from build123d import *

# Parameters (mm, degrees)
BOSS_EXTRUDE1_DEPTH = 3


with BuildPart() as part:
    # Sketch1 → Boss-Extrude1 (new body)
    with BuildSketch(Plane(origin=(0, 0, 0), x_dir=(1, 0, 0), z_dir=(0, 1, 0))):
        Polygon((-5, 44.5), (-25.5, 35.5), (25.5, 35.5), (5, 44.5), align=None)
        Polygon((-25.5, 35.5), (-35.5, 35.5), (-35.5, -35.5), (35.5, -35.5), (35.5, 35.5), (25.5, 35.5), align=None)
    extrude(amount=BOSS_EXTRUDE1_DEPTH)


solid = part.part
Design review of the part built by this model. Coordinates are the model's own, in mm. A direction names the side the tool comes from. Coordinates: 2 decimals unless noted, no trailing zeros. Loops run counter-clockwise (first coordinate to the right, second up) from the corner with the lowest first, then second, coordinate; pieces in that order, holes last. Notation, with made-up numbers: (-31.5, 22) - (-12.5, 22) arc R13 cw to (-12.5, 31) - close; hole circle Ø2 at (56.25, 56). An arc over 180 degrees is marked (long way). Use CSV: the item, a comma, the result in double quotes. Start each with the question number.
1. Add section C-C on z = -38. Give the boundary of the cut face in (x, y), plus the area to 3 significant figures.
2. Clearance check with a flat-ended pin moving along its axis: pin 1 (1.5 mm diameter, centred on x = -29, y = 2, fed in from -Z). State where the tip first meets the part, or that it passes through.
3. Add section A-A on y = 1.2. Give the boundary of the cut face in (x, z), plus the area to 3 significant figures.
4. For faces 1 (the flat face through (0, 3, -5)), 2 (the flat face through (-30, 1, -35.5)), 3 (the flat face through (31, 1, -35.5)), list the 3-axis set-ups (+Z, -Z, +X, -X, +Y, -Y) from which the entire face can be reached by the end or side of a thin tool; tool diameter is ignored.
5. Add section B-B on x = 10. Give the boundary of the cut face in (y, z).
6. To check wall thickness, follow probe 1 along Z at (x, y) = (-32, 1.95); probe 2 along Z at (x, y) = (9, 1.5); probe 3 along X at (y, z) = (0.95, -36). State the ranges of each line that lie inside material, in increasing order.
Resolved:
1,outline,"(-19.81, 0) - (19.81, 0) - (19.81, 3) - (-19.81, 3) - close"
1,area,"119 mm2"
2,pin 1,"z = -35.5"
3,outline,"(-35.5, -35.5) - (-25.5, -35.5) - (-5, -44.5) - (5, -44.5) - (25.5, -35.5) - (35.5, -35.5) - (35.5, 35.5) - (-35.5, 35.5) - close"
3,area,"5,320 mm2"
4,face 1,"+Z, -Z, +X, -X, +Y"
4,face 2,"-Z, -X, +Y, -Y"
4,face 3,"-Z, +X, +Y, -Y"
5,outline,"(0, -42.3) - (3, -42.3) - (3, 35.5) - (0, 35.5) - close"
6,probe 1,"-35.5 to 35.5"
6,probe 2,"-42.74 to 35.5"
6,probe 3,"-24.36 to 24.36"
